from build123d import *

# Parameters (mm, degrees)
F0_W     = 29.265608
F0_H     = 29.265608
F0_R     = 1.8288
F0_R_2   = 9.525
F1_DEPTH = 12.7
F2_R     = 3.96875
F3_R     = 11.1125
F4_DEPTH = 8.89


with BuildPart() as f1:
    # F0 (on Top) → F1 (new body)
    with BuildSketch(Plane.XY):
        Rectangle(F0_W, F0_H)
        with Locations((-10.664054, -10.664054)):
            Circle(F0_R, mode=Mode.SUBTRACT)
        with Locations((10.664054, -10.664054)):
            Circle(F0_R, mode=Mode.SUBTRACT)
        with Locations((-10.664054, 10.664054)):
            Circle(F0_R, mode=Mode.SUBTRACT)
        Circle(F0_R_2, mode=Mode.SUBTRACT)
        with Locations((10.664054, 10.664054)):
            Circle(F0_R, mode=Mode.SUBTRACT)
    extrude(amount=F1_DEPTH)

    # F2
    f2_edges = [f1.edges().sort_by_distance(p)[0] for p in [
        (-14.632804, 14.632804, 6.35),
        (-14.632804, -14.632804, 6.35),
        (14.632804, -14.632804, 6.35),
        (14.632804, 14.632804, 6.35),
    ]]
    fillet(f2_edges, radius=F2_R)

    # F3 (on face) → F4 (cut)
    with BuildSketch(Plane(origin=(0, 0, 0), x_dir=(1, 0, 0), z_dir=(0, 0, -1))):
        Circle(F3_R)
    extrude(amount=-F4_DEPTH, mode=Mode.SUBTRACT)


solid = f1.part
Input: part model. Units: mm. Frame: model coordinates. A direction names the side the tool comes from. Coordinates: 2 decimals unless noted, no trailing zeros. Write each loop counter-clockwise with the first axis right and the second up, starting at its lowest first coordinate (ties: lowest second). Pieces come first, ordered by that corner, then holes. Notation, with made-up numbers: M 43.5,15.25 L 68.5,15.25 A19 ccw 68.5,21.25 Z; hole C 75.25,55.5 d8. An arc over 180 degrees is marked long. Answer as a JSON object with one key per item and string values. Group by question number.
(1) Ray query, line 1 along Y through (x, z) = (9.5, 2.25); line 2 along X through (y, z) = (-11.25, 11.25); line 3 along Y through (x, z) = (0, 5.75). Return the intervals inside material, ascending. Write a range as [from, to].
(2) Section D-D on z = 6.75. Output: boundary loops of the cut face in (x, y) (1 decimal), plus the area to 3 significant figures.
(3) Set-up query: faces 4 (the face through (-7.559, -5.796, 10.768)), 5 (the face through (10.6, -3.34, 4.38)). Return all of +Z, -Z, +X, -X, +Y, -Y with unobstructed straight access to the full face (end or side cutting, diameter ignored); none if empty.
(4) Mould query, pull axis X, two halves, no side actions, for faces 1 (the face through (-13.5, -13.44, 6.44)), 2 (the face through (-5, -8.3, 8.89)), 3 (the face through (0, 10, 12.7)). Classes: pulls with the +X half, pulls with the -X half, needs draft (parallel to the pull), parting line crosses it, or undercut.
(5) Section A-A on y = 0. Output: boundary loops of the cut face in (x, z) (1 decimal).
(6) Section B-B on z = 11. Give the number of separate pieces and of enclosed holes in the cut face, plus the area to 3 significant figures.
Result set:
{
 "1": {"line 1": "y = [-14.63, -12.07], [-9.25, -5.77], [5.77, 9.25], [12.07, 14.63]", "line 2": "x = [-14.59, -12.4], [-8.93, 8.93], [12.4, 14.59]", "line 3": "y = [-14.63, -11.11], [11.11, 14.63]"},
 "2": {"outline": "M -14.6,-10.7 A4 ccw -10.7,-14.6 L 10.7,-14.6 A4 ccw 14.6,-10.7 L 14.6,10.7 A4 ccw 10.7,14.6 L -10.7,14.6 A4 ccw -14.6,10.7 Z; hole C -10.7,-10.7 d3.7; hole C -10.7,10.7 d3.7; hole C 0,0 d22.2; hole C 10.7,-10.7 d3.7; hole C 10.7,10.7 d3.7", "area": "413 mm2"},
 "3": {"face 4": "+Z, -Z", "face 5": "-Z"},
 "4": {"face 1": "pulls with the -X half", "face 2": "undercut", "face 3": "needs draft"},
 "5": {"outline": "M -14.6,0 L -11.1,0 L -11.1,8.9 L -9.5,8.9 L -9.5,12.7 L -14.6,12.7 Z; M 9.5,8.9 L 11.1,8.9 L 11.1,0 L 14.6,0 L 14.6,12.7 L 9.5,12.7 Z"},
 "6": {"separate pieces": "1", "enclosed holes": "5", "area": "516 mm2"}
}
